Drawing for the job (mm, zero at the part's lowest x, y, z). A direction names the side the tool comes from. Give positions to 0.01 mm unless a question says otherwise; leave off trailing zeros. Write each loop counter-clockwise with the first axis right and the second up, starting at its lowest first coordinate (ties: lowest second). Pieces come first, ordered by that corner, then holes. Notation, with made-up numbers: M -4.5,26.5 L 47.5,26.5 A16 ccw 47.5,35.5 Z; hole C 43,76 d9. An arc over 180 degrees is marked long. Write item = value, one per line. Start each with the question number.
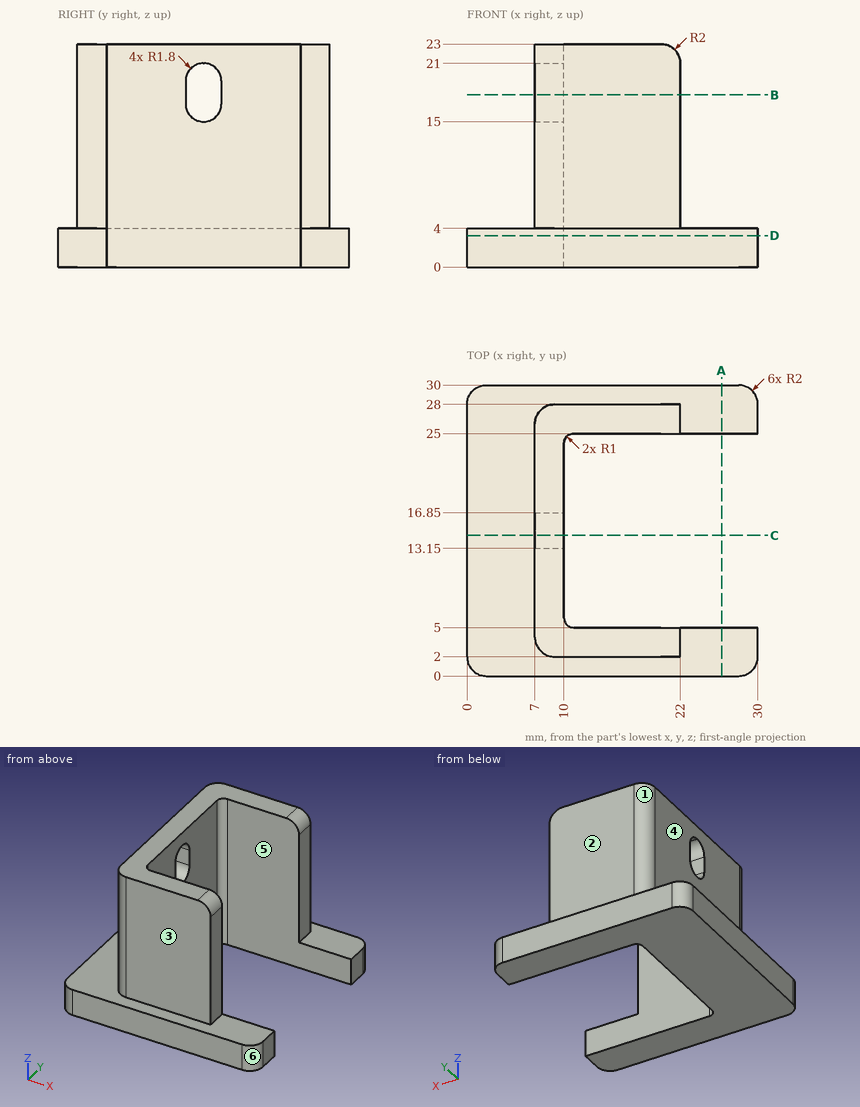
Q1. Slice it at C-C (y = 14.5). Give the cut face in (x, z), and give its area (3 significant figures).
Q2. Probe line 1 along Y through (x, z) = (15.5, 17); line 2 along X through (y, z) = (6.25, 6); line 3 along X through (y, z) = (15.5, 2.75). List the from-to ranges inside material, lowest first.
Q3. Drop flat-ended pins along their axis: P1, Ø6, axis at y = 24.5, z = 3.5, coming from the -X side; P2, Ø1.9, axis at x = 8.5, z = 18.5, coming from the -Y side; P3, Ø1.5, axis at y = 17, z = 12.5, coming from the -X side; P4, Ø3, axis at x = 10, z = 17.5, coming from the +Y side. Give the stop position or say it passes through.
Q4. Slice it at A-A (x = 26.25). Give the cut face in (y, z), and give its area (3 significant figures).
Q5. Slice it at D-D (z = 3.25). Give the cut face in (x, y), and give its area (3 significant figures).
Q6. Tool access for the marked faces 1, 2 and 3: list every direction of +Z, -Z, +X, -X, +Y, -Y with a clear straight run to the whole face (end or side of a thin tool).
Q7. Slice it at B-B (z = 17.75). Give the cut face in (x, y).
Q8. Two-plate mould, pull along Y, no slides. Class the marked faces 4, 5 and 6: +Y half, -Y half, draft (parallel to the pull), parting line (faces both ways), or undercut.
Working result:
q1.outline = M 0,0 L 10,0 L 10,15.06 L 7,15.06 L 7,4 L 0,4 Z; M 7,20.94 L 10,20.94 L 10,23 L 7,23 Z
q1.area = 79.3 mm2
q2.line_1 = 2 to 5, 25 to 28
q2.line_2 = 7 to 10
q2.line_3 = 0 to 10
q3.P1 = 0
q3.P2 = 2
q3.P3 = 7
q3.P4 = 28
q4.outline = M 0,0 L 5,0 L 5,4 L 0,4 Z; M 25,0 L 30,0 L 30,4 L 25,4 Z
q4.area = 40.0 mm2
q5.outline = M 0,2 A2 ccw 2,0 L 28,0 A2 ccw 30,2 L 30,5 L 11,5 A1 cw 10,6 L 10,24 A1 cw 11,25 L 30,25 L 30,28 A2 ccw 28,30 L 2,30 A2 ccw 0,28 Z
q5.area = 497 mm2
q6.face_1 = +Z, -X, +Y
q6.face_2 = +Z, +X, -X, +Y
q6.face_3 = +Z, +X, -X, -Y
q7.outline = M 7,4 A2 ccw 9,2 L 22,2 L 22,5 L 11,5 A1 cw 10,6 L 10,13.15 L 7,13.15 Z; M 7,16.85 L 10,16.85 L 10,24 A1 cw 11,25 L 22,25 L 22,28 L 9,28 A2 ccw 7,26 Z
q8.face_4 = draft
q8.face_5 = undercut
q8.face_6 = -Y half
